The model under review builds one solid part; all positions refer to its coordinate system, in mm. A direction names the side the tool comes from. Round coordinates to 2 decimals unless told otherwise and drop trailing zeros. Write each loop counter-clockwise with the first axis right and the second up, starting at its lowest first coordinate (ties: lowest second). Pieces come first, ordered by that corner, then holes. Notation, with made-up numbers: (-40, -32.75) -> (-30, -32.75) arc R23 cw to (-30, 6.25) -> close; hole circle Ø7 at (60, -39.75). An arc over 180 degrees is marked (long way). Return JSON: item names as keys, results as strings. Group by question number.
1. Mouldability with a two-part tool opening along X and no side actions: class faces 1 (the flat face through (-3.05, -3.61, 11.94)), 2 (the cylindrical face through (2.02, 3.16, 15.28)) as pulls with the +X half, pulls with the -X half, needs draft (parallel to the pull), parting line crosses it, or undercut.
2. Tool access review of faces 3 (the flat face through (-3.05, 3.61, 26.34)), 4 (the flat face through (-1.6, -4, 26)), 5 (the flat face through (4, 2, 14.4)): name each direction out of +Z, -Z, +X, -X, +Y, -Y from which nothing blocks a thin tool from reaching the whole face with its end or side.
3. Take a section at A-A, the plane y = 0. Write out the cut boundary in (x, z), then the cut area to 3 significant figures.
4. Take a section at D-D, the plane x = 0. Give the number of separate pieces and of enclosed holes in the cut face, then the cut area to 3 significant figures.
5. For line 1 along Z through (x, y) = (-3.5, 3.75); line 2 along X through (y, z) = (-4.5, 26); line 3 along Y through (x, z) = (-3.25, 21.5), list the stretches that pass through material, from the lowest coordinate up. Write a range as from..to.
6. Take a section at B-B, the plane z = 12.5. Write out the cut boundary in (x, y).
7. Clearance check with flat-ended pins moving along their axes: P1, Ø5, axis at y = -3, z = 8.5, coming from the -X side; P2, Ø1.7, axis at y = -4.5, z = 11.5, coming from the -X side; P3, Ø1.1, axis at y = -4.5, z = 26.5, coming from the +X side. State where each tip first meets the part, or that it passes through.
8. Take a section at C-C, the plane z = 23.5. Write out the cut boundary in (x, y), then the cut area to 3 significant figures.
from build123d import *

# Parameters (mm, degrees)
SKETCH_1_R               = 5.75
SKETCH_1_R_2             = 4.75
SKETCH_1_R_3             = 3.75
EXTRUDE_1_DEPTH          = 31
SKETCH_2_W               = 3.2
SKETCH_2_H               = 5
CUT_EXTRUDE_1_DEPTH      = 33.048790929
PATTERN_CIRCULAR_1_COUNT = 3


with BuildPart() as part:
    # 草图1 → 凸台-拉伸1 (new body)
    # profile 1 of 2: a face of its own
    with BuildSketch(Plane.XY):
        Circle(SKETCH_1_R)
        Circle(SKETCH_1_R_2, mode=Mode.SUBTRACT)
    # profile 2 of 2: a face of its own
    with BuildSketch(Plane.XY):
        Circle(SKETCH_1_R_2)
        Circle(SKETCH_1_R_3, mode=Mode.SUBTRACT)
    extrude(amount=EXTRUDE_1_DEPTH)

    # 草图2 → 切除-拉伸1 (cut, symmetric)
    with BuildSketch(Plane(origin=(0, 0, 0), x_dir=(1, 0, 0), z_dir=(0, 1, 0))):
        with Locations((0, -4.7)):
            Rectangle(SKETCH_2_W, SKETCH_2_H)
        with Locations((0, -11.9)):
            Rectangle(SKETCH_2_W, SKETCH_2_H)
        with Locations((0, -19.1)):
            Rectangle(SKETCH_2_W, SKETCH_2_H)
        with Locations((0, -26.3)):
            Rectangle(SKETCH_2_W, SKETCH_2_H)
    cut_extrude_1 = extrude(amount=CUT_EXTRUDE_1_DEPTH, both=True, mode=Mode.SUBTRACT)

    # 阵列(圆周)1: 切除-拉伸1 ×3 about axis
    pattern_circular_1_axis = Axis((0, 0, 0), (0, 0, 1))
    for i in range(1, PATTERN_CIRCULAR_1_COUNT):
        add(cut_extrude_1.rotate(pattern_circular_1_axis, i * 360 / PATTERN_CIRCULAR_1_COUNT), mode=Mode.SUBTRACT)


solid = part.part
Output:
{
 "1": {"face 1": "pulls with the -X half", "face 2": "undercut"},
 "2": {"face 3": "-X", "face 4": "+Y, -Y", "face 5": "none"},
 "3": {"outline": "(-5.75, 0) -> (-3.75, 0) -> (-3.75, 31) -> (-5.75, 31) -> close; (3.75, 0) -> (5.75, 0) -> (5.75, 31) -> (3.75, 31) -> close", "area": "124 mm^2"},
 "4": {"separate pieces": "10", "enclosed holes": "0", "area": "44.0 mm^2"},
 "5": {"line 1": "z = 0..2.2, 7.2..9.4, 14.4..16.6, 21.6..23.8, 28.8..31", "line 2": "x = -3.58..-1.6, 1.6..3.58", "line 3": "y = -4.74..-3.72, 3.72..4.74"},
 "6": {"outline": "(-5.58, -1.38) -> (-3.74, -0.31) arc R3.75 cw to (-3.74, 0.31) -> (-5.58, 1.38) arc R5.75 ccw to start; (-3.98, -4.15) arc R5.75 ccw to (-1.6, -5.52) -> (-1.6, -3.39) arc R3.75 cw to (-2.14, -3.08) -> close; (-3.98, 4.15) -> (-2.14, 3.08) arc R3.75 cw to (-1.6, 3.39) -> (-1.6, 5.52) arc R5.75 ccw to start; (1.6, -5.52) arc R5.75 ccw to (3.98, -4.15) -> (2.14, -3.08) arc R3.75 cw to (1.6, -3.39) -> close; (1.6, 3.39) arc R3.75 cw to (2.14, 3.08) -> (3.98, 4.15) arc R5.75 ccw to (1.6, 5.52) -> close; (3.74, -0.31) -> (5.58, -1.38) arc R5.75 ccw to (5.58, 1.38) -> (3.74, 0.31) arc R3.75 cw to start"},
 "7": {"P1": "stops at x = -5.73", "P2": "stops at x = -3.98", "P3": "stops at x = 3.98"},
 "8": {"outline": "circle Ø11.5 at (0, 0); hole circle Ø7.5 at (0, 0)", "area": "59.7 mm^2"}
}
